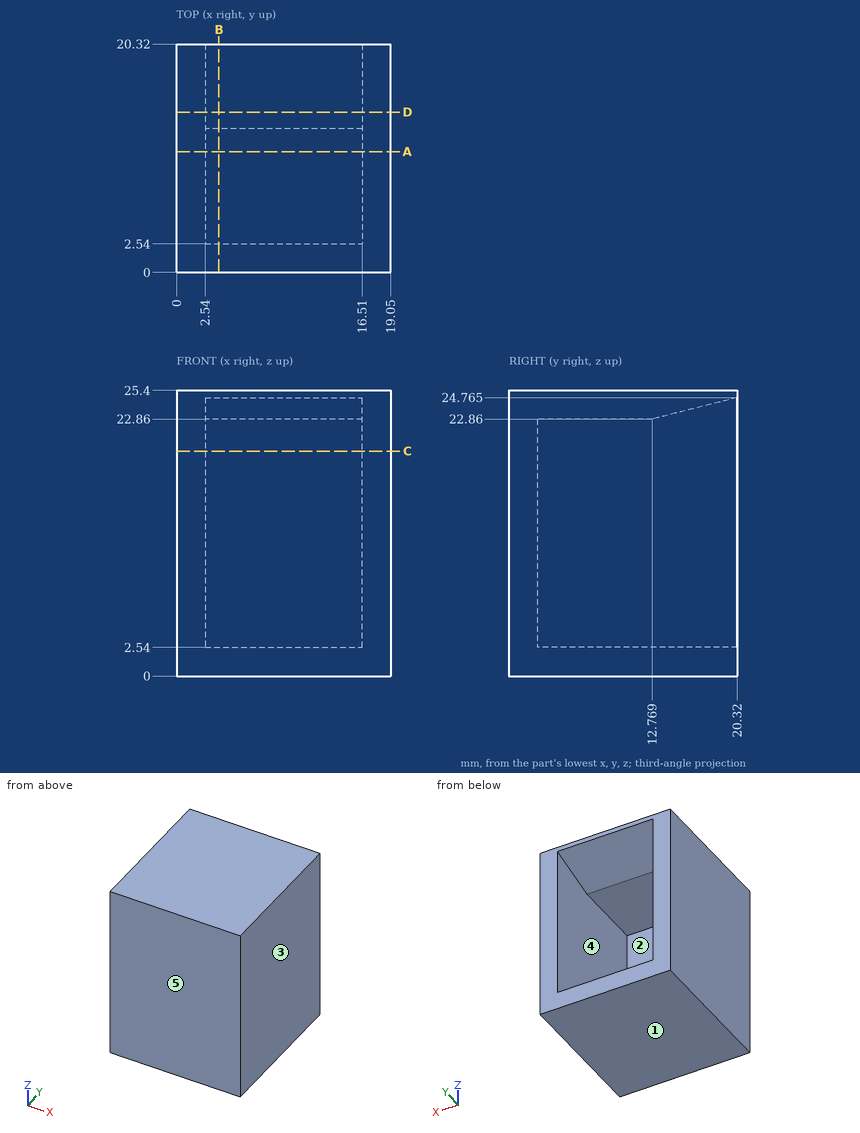
Input: dimensioned drawing with shaded views. Units: mm. Origin: part minimum x, y, z. A direction names the side the tool comes from. Round coordinates to 2 decimals unless told otherwise and drop trailing zeros. Loops run counter-clockwise (first coordinate to the right, second up) from the corner with the lowest first, then second, coordinate; pieces in that order, holes last. Notation, with made-up numbers: M -40,28 L -31,28 A26 cw -31,44 Z; hole C -37.5,88 d5. An arc over 180 degrees is marked long. Return JSON: item names as keys, results as strings. Group by question number.
1. Mould query, pull axis Z, two halves, no side actions, for the marked faces 1, 2 and 3. Classes: released by +Z, released by -Z, zero draft, split by the parting line, or undercut.
2. Material intervals for line 1 along X through (y, z) = (8, 8.5); line 2 along Z through (x, y) = (15.5, 4.25); line 3 along Y through (x, z) = (9.5, 8), sorted ascending. Write a range as from..to.
3. Pin query (flat end, axial travel): pin 1 (4 mm diameter, centred on y = 12.5, z = 13, fed in from -X). Return the tip coordinate at first contact, or that it passes through.
4. Section query A-A on y = 10.75. Output: boundary loops of the cut face in (x, z).
5. Section query C-C on z = 20. Output: boundary loops of the cut face in (x, y).
6. Reachability of the marked faces 4 and 5 from +Z, -Z, +X, -X, +Y, -Y: full face, straight path, thin tool, end or side. Return the list, or none.
7. Section query B-B on x = 3.75. Output: boundary loops of the cut face in (y, z) (1 decimal), and give its area (3 significant figures).
8. Section query D-D on y = 14.25. Output: boundary loops of the cut face in (x, z), and give its area (3 significant figures).
Checks:
{
 "1": {"face 1": "released by -Z", "face 2": "undercut", "face 3": "zero draft"},
 "2": {"line 1": "x = 0..2.54, 16.51..19.05", "line 2": "z = 0..2.54, 22.86..25.4", "line 3": "y = 0..2.54"},
 "3": {"pin 1": "stops at x = 0"},
 "4": {"outline": "M 0,0 L 19.05,0 L 19.05,25.4 L 0,25.4 Z; hole M 2.54,2.54 L 16.51,2.54 L 16.51,22.86 L 2.54,22.86 Z"},
 "5": {"outline": "M 0,0 L 19.05,0 L 19.05,20.32 L 16.51,20.32 L 16.51,2.54 L 2.54,2.54 L 2.54,20.32 L 0,20.32 Z"},
 "6": {"face 4": "+Y", "face 5": "+Z, -Z, +X, -X, -Y"},
 "7": {"outline": "M 0,0 L 20.3,0 L 20.3,2.5 L 2.5,2.5 L 2.5,22.9 L 12.8,22.9 L 20.3,24.8 L 20.3,25.4 L 0,25.4 Z", "area": "148 mm²"},
 "8": {"outline": "M 0,0 L 19.05,0 L 19.05,25.4 L 0,25.4 Z; hole M 2.54,2.54 L 16.51,2.54 L 16.51,23.23 L 2.54,23.23 Z", "area": "195 mm²"}
}
